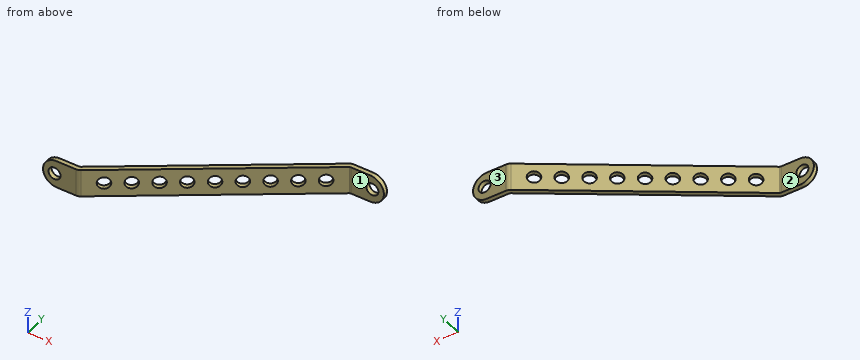
from build123d import *

# Parameters (mm, degrees)
EXTRUDE_THIN1_DEPTH = 4.8
SKETCH2_R           = 2.1
CUT_EXTRUDE1_DEPTH  = 100.04584797
SKETCH3_R           = 2.1
CUT_EXTRUDE2_DEPTH  = 100.786171387
FILLET1_R           = 4.8
SKETCH4_R           = 2.1
CUT_EXTRUDE3_DEPTH  = 99.787603571
LPATTERN1_COUNT     = 5
LPATTERN1_PITCH     = 8
LPATTERN2_COUNT     = 5
LPATTERN2_PITCH     = 8


with BuildPart() as part:
    # Sketch1 → Extrude-Thin1 (new body)
    with BuildSketch(Plane.XY):
        with BuildLine():
            Line((0, -0.8), (11.491963677, -0.8))
            ThreePointArc((11.491963677, -0.8), (12.218283231, -0.687457083), (12.87648435, -0.360383255))
            Line((12.87648435, -0.360383255), (76.046529432, 44.253461085))
            ThreePointArc((76.046529432, 44.253461085), (76.265929805, 44.362485694), (76.508036323, 44.4))
            Line((76.508036323, 44.4), (88, 44.4))
            Line((88, 44.4), (88, 46))
            Line((88, 46), (76.508036323, 46))
            ThreePointArc((76.508036323, 46), (75.781716769, 45.887457083), (75.12351565, 45.560383255))
            Line((75.12351565, 45.560383255), (11.953470568, 0.946538915))
            ThreePointArc((11.953470568, 0.946538915), (11.734070195, 0.837514306), (11.491963677, 0.8))
            Line((11.491963677, 0.8), (0, 0.8))
            Line((0, 0.8), (0, -0.8))
        make_face()
    extrude(amount=EXTRUDE_THIN1_DEPTH)

    # Sketch2 → Cut-Extrude1 (cut, through all)
    with BuildSketch(Plane(origin=(0, 0.8, 0), x_dir=(1, 0, 0), z_dir=(0, 1, 0))):
        with Locations((4, 0)):
            Circle(SKETCH2_R)
    extrude(amount=-CUT_EXTRUDE1_DEPTH, mode=Mode.SUBTRACT)

    # Sketch3 → Cut-Extrude2 (cut, through all)
    with BuildSketch(Plane(origin=(0, 46, 0), x_dir=(1, 0, 0), z_dir=(0, 1, 0))):
        with Locations((84, 0)):
            Circle(SKETCH3_R)
    extrude(amount=-CUT_EXTRUDE2_DEPTH, mode=Mode.SUBTRACT)

    # Fillet1
    fillet1_edges = [part.edges().sort_by_distance(p)[0] for p in [
        (0, 0, 4.8),
        (88, 45.2, 4.8),
    ]]
    fillet(fillet1_edges, radius=FILLET1_R - 0.0001)  # a hair under: the kernel refuses the full size

    # Sketch4 → Cut-Extrude3 (cut, through all)
    with BuildSketch(Plane(origin=(3.532029558, -5.001103798, 0), x_dir=(0.816826356052519, 0.5768836139620918, 0), z_dir=(-0.5768836139620916, 0.8168263560525189, 0))):
        with Locations((48.977929342, 0)):
            Circle(SKETCH4_R)
    cut_extrude3 = extrude(amount=-CUT_EXTRUDE3_DEPTH, mode=Mode.SUBTRACT)

    # LPattern1: Cut-Extrude3 ×5
    with Locations(*[Vector(0.8168263560525189, 0.5768836139620918, 0) * (i * LPATTERN1_PITCH) for i in range(1, LPATTERN1_COUNT)]):
        add(cut_extrude3, mode=Mode.SUBTRACT)

    # LPattern2: Cut-Extrude3 ×5
    with Locations(*[Vector(-0.8168263560525189, -0.5768836139620918, 0) * (i * LPATTERN2_PITCH) for i in range(1, LPATTERN2_COUNT)]):
        add(cut_extrude3, mode=Mode.SUBTRACT)

    # Mirror1: part across plane


with BuildPart() as part_1:
    add(part.part)
    add(part.part.mirror(Plane(origin=(76.508036323, 43.6, 0), x_dir=(1, 0, 0), z_dir=(0, 0, 1))))


solid = part_1.part
Part model, mm, in its own coordinate system. Face numbers are marked on the shaded views. A direction names the side the tool comes from. Coordinates: 2 decimals unless noted, no trailing zeros. Order: outer loops, then holes, each group sorted by start corner. A loop starts at its lowest first (then second) coordinate and runs counter-clockwise, first axis right, second up.
(1) Pin check, flat tips, straight feed: pin 1 Ø5.5 at (x, z) = (4, 0) entering from +Y; pin 2 Ø2 at (y, z) = (33, 0.5) entering from +X; pin 3 Ø3 at (y, z) = (31.5, -4) entering from +X. Stop position of each tip, or through.
Check sheet entries:
pin 1: stops at y = 0.8
pin 2: stops at x = 61.53
pin 3: stops at x = 60.11
(2) Slice it at B-B, the plane x = 80.5. Write the cut outline in (y, z), and give its area (3 significant figures).
Check sheet entries:
outline: (44.4, -4.8) - (46, -4.8) - (46, 4.8) - (44.4, 4.8) - close
area: 15.4 mm2
(3) Tool access for the marked faces 1, 2 and 3: list every direction of +Z, -Z, +X, -X, +Y, -Y with a clear straight run to the whole face (end or side of a thin tool).
Check sheet entries:
face 1: +Z, -Z, +X, -Y
face 2: +Z, -Z, -X, +Y
face 3: +Z, -Z, +X, -X, +Y
(4) Slice it at A-A, the plane z = -3.75. Write the cut outline in (x, y).
Check sheet entries:
outline: (1.8, -0.8) - (11.49, -0.8) arc R2.4 ccw to (12.88, -0.36) - (76.05, 44.25) arc R0.8 cw to (76.51, 44.4) - (86.2, 44.4) - (86.2, 46) - (76.51, 46) arc R2.4 ccw to (75.12, 45.56) - (11.95, 0.95) arc R0.8 cw to (11.49, 0.8) - (1.8, 0.8) - close
(5) Probe L1, parallel to Z at x = 4, y = -0.15; L2, parallel to Y at x = 5.5, z = 4.75; L3, parallel to Y at x = 80, z = -2.5. List the from-to ranges inside material, lowest first.
Check sheet entries:
L1: z = -4.73 to -2.1, 2.1 to 4.73
L2: y = -0.8 to 0.8
L3: y = 44.4 to 46
